Check sheet for the modelled part. Datum: model origin and axes. Units: mm. A direction names the side the tool comes from. Give positions to 0.01 mm unless a question says otherwise; leave off trailing zeros. Loops run counter-clockwise (first coordinate to the right, second up) from the corner with the lowest first, then second, coordinate; pieces in that order, holes last. Notation, with made-up numbers: (10.5, 42.5) - (15.5, 42.5) arc R16 ccw to (15.5, 56.5) - close; hole circle Ø4 at (-6, 17). An arc over 180 degrees is marked (long way). Answer in a Markdown table with one row per item. Add a question column.
(1) Draft check along Y on faces 1 (the face through (6, 28.937, -19)), 2 (the face through (6, -5, -18.137)), 3 (the face through (-9, 10, -6.137)). Enter one of: released by +Y, released by -Y, zero draft, split by the parting line, or undercut.
(2) Go/stop test with flat-tipped pins: P1, Ø8, axis at y = -6, z = -12.5, coming from the +X side; P2, Ø2, axis at x = 23, z = -13.5, coming from the +Y side; P3, Ø4, axis at y = 25, z = -12, coming from the +X side. Record where each tip stops, or that it passes through.
(3) Sectioned sample at D-D on x = 6. Enter the section's corners in (y, z).
(4) Sectioned sample at B-B on z = -15. Enter the section's corners in (x, y).
(5) Sectioned sample at C-C on z = -4.5. Enter the section's corners in (x, y), then the cut area to 3 significant figures.
(6) Sectioned sample at A-A on y = 10. Enter the section's corners in (x, z).
(7) Set-up check for faces 4 (the face through (14, 14, -6.937)), 5 (the face through (6, 21.437, -12)), 6 (the face through (-9, 16, -12)): record each of +Z, -Z, +X, -X, +Y, -Y from which the full face is reachable in a straight line by a thin tool's end or side.
(8) Thickness scan on L1, parallel to X at y = 10, z = -7.15; L2, parallel to X at y = 10, z = -4.65; L3, parallel to Z at x = 23, y = 12. Record the ranges inside material, lowest first.
from build123d import *

# Parameters (mm, degrees)
SKIZZE1_W                          = 37.873435046
SKIZZE1_H                          = 37.873435047
AUFSATZ_LINEAR_AUSTRAGEN1_DEPTH    = 20
SKIZZE2_R                          = 10.55
SCHNITT_LINEAR_AUSTRAGEN1_DEPTH    = 4
SKIZZE3_W                          = 12
SKIZZE3_H                          = 12
SCHNITT_LINEAR_AUSTRAGEN3_DEPTH    = 7.5
VERRUNDUNG1_R                      = 8
KREISMUSTER1_COUNT                 = 4
SKIZZE4_R                          = 8.75
SCHNITT_LINEAR_AUSTRAGEN4_DEPTH    = 0.5
K_RPER_VERSCHIEBEN_KOPIEREN1_ANGLE = 90


with BuildPart() as part:
    # Skizze1 → Aufsatz-Linear austragen1 (new body)
    with BuildSketch(Plane(origin=(0, 0, 0), x_dir=(1, 0, 0), z_dir=(0, 1, 0))):
        with Locations((6, 12.936717524)):
            Rectangle(SKIZZE1_W, SKIZZE1_H)
    extrude(amount=AUFSATZ_LINEAR_AUSTRAGEN1_DEPTH)

    # Skizze2 → Schnitt-Linear austragen1 (cut)
    with BuildSketch(Plane.XZ):
        with Locations(Location((6, -12.936717523, 0), (0, 0, 270))):
            Circle(SKIZZE2_R)
    extrude(amount=-SCHNITT_LINEAR_AUSTRAGEN1_DEPTH, mode=Mode.SUBTRACT)

    # Skizze3 → Schnitt-Linear austragen3 (cut)
    with BuildSketch(Plane.XY.offset(6)):
        with Locations((6, 9.2)):
            Rectangle(SKIZZE3_W, SKIZZE3_H)
    schnitt_linear_austragen3 = extrude(amount=-SCHNITT_LINEAR_AUSTRAGEN3_DEPTH, mode=Mode.SUBTRACT)

    # Verrundung1
    verrundung1_edges = [part.edges().sort_by_distance(p)[0] for p in [
        (24.936717523, 10, -31.873435047),
        (24.936717523, 10, 6),
        (-12.936717523, 10, 6),
        (-12.936717523, 10, -31.873435047),
    ]]
    fillet(verrundung1_edges, radius=VERRUNDUNG1_R)

    # Kreismuster1: Schnitt-Linear austragen3 ×4 about axis
    kreismuster1_axis = Axis((6, 0, -12.936717523), (0, 1, 0))
    for i in range(1, KREISMUSTER1_COUNT):
        add(schnitt_linear_austragen3.rotate(kreismuster1_axis, i * 360 / KREISMUSTER1_COUNT), mode=Mode.SUBTRACT)

    # Skizze4 → Schnitt-Linear austragen4 (cut)
    with BuildSketch(Plane.XZ.offset(-4)):
        with Locations(Location((6, -12.936717523, 0), (0, 0, 270))):
            Circle(SKIZZE4_R)
    extrude(amount=-SCHNITT_LINEAR_AUSTRAGEN4_DEPTH, mode=Mode.SUBTRACT)


with BuildPart() as part_1:
    # Körper-Verschieben/Kopieren1: moved
    add(part.part.rotate(Axis((0, 10, -12.936717523), (-1, 0, 0)), K_RPER_VERSCHIEBEN_KOPIEREN1_ANGLE))


solid = part_1.part
Reply:
| question | item | result |
|---|---|---|
| 1 | face 1 | released by +Y |
| 1 | face 2 | zero draft |
| 1 | face 3 | undercut |
| 2 | P1 | x = 24.87 |
| 2 | P2 | y = 27.13 |
| 2 | P3 | x = 24.67 |
| 3 | outline | (-8.94, -22.94) - (28.94, -22.94) - (28.94, -18.14) - (21.44, -18.14) - (21.44, -6.14) - (28.94, -6.14) - (28.94, -2.94) - (20.55, -2.94) - (20.55, -6.94) - (18.75, -6.94) - (18.75, -7.44) - (1.25, -7.44) - (1.25, -6.94) - (-0.55, -6.94) - (-0.55, -2.94) - (-8.94, -2.94) - (-8.94, -6.14) - (-1.44, -6.14) - (-1.44, -18.14) - (-8.94, -18.14) - close |
| 4 | outline | (-12.94, -0.94) arc R8 ccw to (-4.94, -8.94) - (0, -8.94) - (0, -1.44) - (12, -1.44) - (12, -8.94) - (16.94, -8.94) arc R8 ccw to (24.94, -0.94) - (24.94, 4) - (17.44, 4) - (17.44, 16) - (24.94, 16) - (24.94, 20.94) arc R8 ccw to (16.94, 28.94) - (12, 28.94) - (12, 21.44) - (0, 21.44) - (0, 28.94) - (-4.94, 28.94) arc R8 ccw to (-12.94, 20.94) - (-12.94, 16) - (-5.44, 16) - (-5.44, 4) - (-12.94, 4) - close |
| 5 | outline | (-12.94, -0.94) arc R8 ccw to (-4.94, -8.94) - (16.94, -8.94) arc R8 ccw to (24.94, -0.94) - (24.94, 20.94) arc R8 ccw to (16.94, 28.94) - (-4.94, 28.94) arc R8 ccw to (-12.94, 20.94) - close; hole circle Ø21.1 at (6, 10) |
| 5 | area | 1,030 mm^2 |
| 6 | outline | (-12.94, -22.94) - (24.94, -22.94) - (24.94, -18.14) - (17.44, -18.14) - (17.44, -6.14) - (24.94, -6.14) - (24.94, -2.94) - (16.55, -2.94) - (16.55, -6.94) - (14.75, -6.94) - (14.75, -7.44) - (-2.75, -7.44) - (-2.75, -6.94) - (-4.55, -6.94) - (-4.55, -2.94) - (-12.94, -2.94) - (-12.94, -6.14) - (-5.44, -6.14) - (-5.44, -18.14) - (-12.94, -18.14) - close |
| 7 | face 4 | +Z |
| 7 | face 5 | +Y |
| 7 | face 6 | -X |
| 8 | L1 | -5.44 to -2.75, 14.75 to 17.44 |
| 8 | L2 | -12.94 to -4.55, 16.55 to 24.94 |
| 8 | L3 | -22.94 to -18.14, -6.14 to -2.94 |
